The listing builds one solid part. Answer for the finished solid, in the listing's coordinates (mm). Face numbers are marked on the shaded views. A direction names the side the tool comes from. Round coordinates to 2 decimals unless told otherwise and drop trailing zeros. Loops run counter-clockwise (first coordinate to the right, second up) from the corner with the lowest first, then second, coordinate; pieces in that order, holes last. Notation, with made-up numbers: M -2.5,16 L 43.5,16 A23 ccw 43.5,50 Z; hole C 2,44 d2. An arc over 180 degrees is marked long. Put each result on its own line as item: value. Start each with the question number.
(1) Which of the six approach directions +Z, -Z, +X, -X, +Y, -Y give full straight-line access (tool end or side, diameter ignored) to the marked faces 1 and 2?
(2) Flat-ended cylindrical pins translate along their axes: P1, Ø10, axis at y = 31, z = 7.5, coming from the -X side; P2, Ø5, axis at x = -26, y = 25, coming from the -Z side; P3, Ø10, axis at x = -10, y = 37, coming from the -Z side. Find the tip coordinate at first contact, or state that the pin passes through.
(3) Straight lines are drawn through the part: line 1 (Y direction, x = -23, z = 16); line 2 (Y direction, x = 17, z = -45.5); line 3 (Z direction, x = 1, y = 10.5). For each, find the intervals that lie inside material, in ascending order.
(4) Section D-D, the plane z = 19.5 is taken. Determine the outline of the cut face in (x, y).
(5) Section A-A, the plane x = 0 is taken. Determine the outline of the cut face in (y, z).
(6) Section B-B, the plane z = 0 is taken. Determine the outline of the cut face in (x, y).
(7) Section C-C, the plane y = -6.5 is taken. Determine the outline of the cut face in (x, z), then the cut area to 3 significant figures.
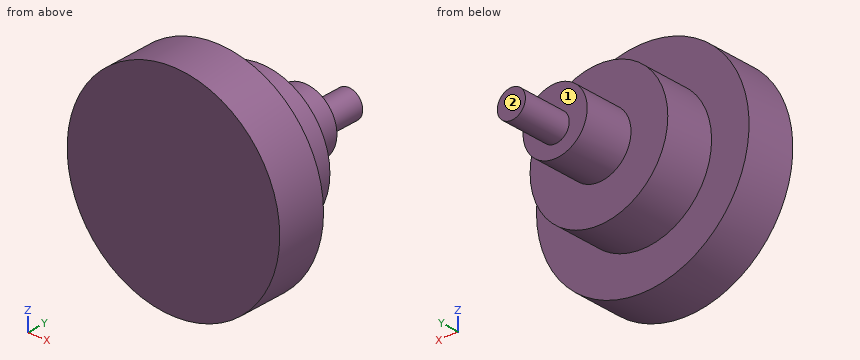
```python
from build123d import *

# Parameters (mm, degrees)
F0_R     = 54.15088
F1_DEPTH = 25.4
F2_R     = 35.080645
F3_DEPTH = 25.4
F4_R     = 16.327777
F5_DEPTH = 25.4
F6_R     = 7.16725
F7_DEPTH = 25.4


with BuildPart() as f1:
    # F0 (on Front) → F1 (new body)
    with BuildSketch(Plane.XZ):
        Circle(F0_R)
    extrude(amount=F1_DEPTH)

    # F2 (on face) → F3 (join)
    with BuildSketch(Plane(origin=(0, 0, 0), x_dir=(-1, 0, 0), z_dir=(0, 1, 0))):
        Circle(F2_R)
    extrude(amount=F3_DEPTH)

    # F4 (on face) → F5 (join)
    with BuildSketch(Plane(origin=(0, 25.4, 0), x_dir=(-1, 0, 0), z_dir=(0, 1, 0))):
        Circle(F4_R)
    extrude(amount=F5_DEPTH)

    # F6 (on face) → F7 (join)
    with BuildSketch(Plane(origin=(0, 50.8, 0), x_dir=(-1, 0, 0), z_dir=(0, 1, 0))):
        with Locations((0, -2.772863)):
            Circle(F6_R)
    extrude(amount=F7_DEPTH)


solid = f1.part
```
Recorded:
1. face 1: +Y
1. face 2: +Z, -Z, +X, -X, +Y
2. P1: stops at x = -16.14
2. P2: stops at z = -26.05
2. P3: stops at z = -15.54
3. line 1: y = -25.4 to 25.4
3. line 2: y = -25.4 to 0
3. line 3: z = -35.07 to 35.07
4. outline: M -50.52,-25.4 L 50.52,-25.4 L 50.52,0 L 29.16,0 L 29.16,25.4 L -29.16,25.4 L -29.16,0 L -50.52,0 Z
5. outline: M -25.4,-54.15 L 0,-54.15 L 0,-35.08 L 25.4,-35.08 L 25.4,-16.33 L 50.8,-16.33 L 50.8,-9.94 L 76.2,-9.94 L 76.2,4.39 L 50.8,4.39 L 50.8,16.33 L 25.4,16.33 L 25.4,35.08 L 0,35.08 L 0,54.15 L -25.4,54.15 Z
6. outline: M -54.15,-25.4 L 54.15,-25.4 L 54.15,0 L 35.08,0 L 35.08,25.4 L 16.33,25.4 L 16.33,50.8 L 6.61,50.8 L 6.61,76.2 L -6.61,76.2 L -6.61,50.8 L -16.33,50.8 L -16.33,25.4 L -35.08,25.4 L -35.08,0 L -54.15,0 Z
7. outline: C 0,0 d108.3
7. area: 9,210 mm²
